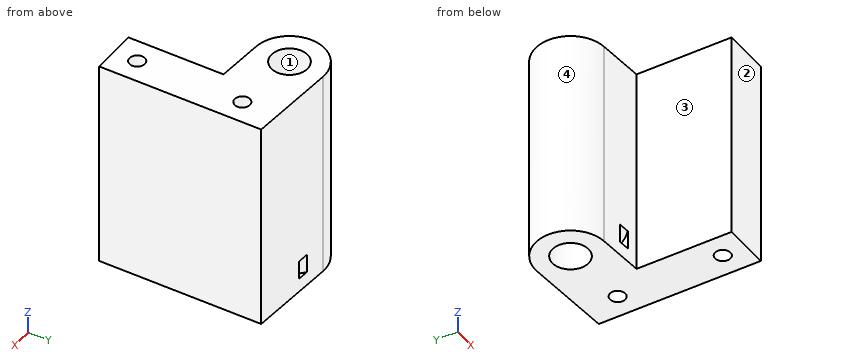
```python
from build123d import *

# Parameters (mm, degrees)
BOSS_EXTRUDE1_DEPTH   = 45
CUT_EXTRUDE1_START    = -5
CUT_EXTRUDE1_DEPTH    = 2
M4X0_7_TAPPED_HOLE1_D = 3.3
SKETCH5_R             = 7.5
BOSS_EXTRUDE2_DEPTH   = 45
SKETCH6_R             = 3.875
CUT_EXTRUDE2_DEPTH    = 46


with BuildPart() as part:
    # Sketch1 → Boss-Extrude1 (new body)
    with BuildSketch(Plane.XY):
        with BuildLine():
            Line((-182.516015687, 162.517772537), (-172.5, 161.827012834))
            Line((-172.5, 161.827012834), (-172.5, 141.5))
            Line((-172.5, 141.5), (-162.5, 141.5))
            Line((-162.5, 141.5), (-162.5, 176.172987166))
            Line((-162.5, 176.172987166), (-181.483984313, 177.482227463))
            ThreePointArc((-181.483984313, 177.482227463), (-174.517772537, 169.483984313), (-182.516015687, 162.517772537))
        make_face()
    extrude(amount=BOSS_EXTRUDE1_DEPTH)

    # Sketch2 → Cut-Extrude1 (cut, symmetric)
    with BuildSketch(Plane(origin=(0, 0, 0), x_dir=(-1, 0, 0), z_dir=(0, 0, -1)).offset(CUT_EXTRUDE1_START)):
        with BuildLine():
            ThreePointArc((176.520836095, 177.139941379), (173.021327044, 169.380781175), (177.552867469, 162.175486453))
            ThreePointArc((177.552867469, 162.175486453), (177.834315887, 161.15284928), (176.811678714, 160.871400862))
            ThreePointArc((176.811678714, 160.871400862), (171.524881552, 169.277578038), (175.60764211, 178.329931609))
            ThreePointArc((175.60764211, 178.329931609), (176.659234217, 178.191533486), (176.520836095, 177.139941379))
        make_face()
    extrude(amount=CUT_EXTRUDE1_DEPTH, both=True, mode=Mode.SUBTRACT)

    # M4x0.7 Tapped Hole1 (through all)
    with Locations(Plane.XY.offset(45)):
        with Locations((-167.5, 169), (-167.5, 146.5)):
            Hole(M4X0_7_TAPPED_HOLE1_D / 2)

    # Sketch5 → Boss-Extrude2 (add, through all)
    with BuildSketch(Plane.XY.offset(45)):
        with Locations((-182, 170)):
            Circle(SKETCH5_R)
    extrude(amount=-BOSS_EXTRUDE2_DEPTH)

    # Sketch6 → Cut-Extrude2 (cut, through all)
    with BuildSketch(Plane.XY.offset(45)):
        with Locations((-182, 170)):
            Circle(SKETCH6_R)
    extrude(amount=-CUT_EXTRUDE2_DEPTH, mode=Mode.SUBTRACT)


solid = part.part
```
For this review, take the finished solid that the model builds, in its own axes (mm). Face numbers are marked on the shaded views. Coordinates: 2 decimals unless noted, no trailing zeros. Loops run counter-clockwise (first coordinate to the right, second up) from the corner with the lowest first, then second, coordinate; pieces in that order, holes last. Notation, with made-up numbers: (-17.5, 62) -> (-9.5, 62) arc R21 cw to (-9.5, 93) -> close; hole circle Ø2 at (67, 20). An arc over 180 degrees is marked (long way). Return JSON: item names as keys, results as strings. Group by question number.
(1) Consider section A-A, the plane y = 169. Give the boundary of the cut face in (x, z), plus the area to 3 significant figures.
(2) Consider section D-D, the plane y = 164. Give the boundary of the cut face in (x, z).
(3) Consider section B-B, the plane x = -182. Give the boundary of the cut face in (y, z) (3 decimals), plus the area to 3 significant figures.
(4) Consider section C-C, the plane z = 8. Give the boundary of the cut face in (x, y) (3 decimals), plus the area to 3 significant figures.
(5) For pin 1 Ø4 at (x, z) = (-181.5, 24) entering from -Y; pin 2 Ø3 at (x, y) = (-167.5, 146.5) entering from +Z; pin 3 Ø16.5 at (y, z) = (156.5, 18.5) entering from -X; pin 4 Ø5 at (x, z) = (-171.5, 25.5) entering from +Y, all flat-tipped, find the tip position at first contact; note any pin that passes through.
(6) To check wall thickness, follow L1, parallel to Y at x = -168.75, z = 6; L2, parallel to X at y = 146.5, z = 26.5; L3, parallel to Y at x = -167.5, z = 30. State the ranges of each line that lie inside material, in increasing order.
(7) Mouldability with a two-part tool opening along Y and no side actions: class the marked faces 1, 2, 3 and 4 as pulls with the +Y half, pulls with the -Y half, needs draft (parallel to the pull), parting line crosses it, or undercut.
Results below:
{
 "1": {"outline": "(-189.43, 0) -> (-185.74, 0) -> (-185.74, 45) -> (-189.43, 45) -> close; (-178.26, 0) -> (-169.15, 0) -> (-169.15, 45) -> (-178.26, 45) -> close; (-165.85, 0) -> (-162.5, 0) -> (-162.5, 45) -> (-165.85, 45) -> close; hole (-173.06, 3) -> (-171.55, 3) -> (-171.55, 7) -> (-173.06, 7) -> close", "area": "721 mm2"},
 "2": {"outline": "(-186.5, 0) -> (-162.5, 0) -> (-162.5, 45) -> (-186.5, 45) -> close; hole (-175.29, 3) -> (-173.38, 3) -> (-173.38, 7) -> (-175.29, 7) -> close"},
 "3": {"outline": "(162.482, 0) -> (166.125, 0) -> (166.125, 45) -> (162.482, 45) -> close; (173.875, 0) -> (177.5, 0) -> (177.5, 45) -> (173.875, 45) -> close", "area": "327 mm2"},
 "4": {"outline": "(-182.516, 162.518) -> (-172.5, 161.827) -> (-172.5, 141.5) -> (-162.5, 141.5) -> (-162.5, 176.173) -> (-181.484, 177.482) arc R7.5 ccw to start; hole circle Ø7.75 at (-182, 170); hole circle Ø3.3 at (-167.5, 146.5); hole circle Ø3.3 at (-167.5, 169)", "area": "517 mm2"},
 "5": {"pin 1": "stops at y = 162.31", "pin 2": "passes through", "pin 3": "stops at x = -187.36", "pin 4": "stops at y = 176.97"},
 "6": {"L1": "y = 141.5 to 145.42, 147.58 to 167.92, 170.08 to 176.6", "L2": "x = -172.5 to -169.15, -165.85 to -162.5", "L3": "y = 141.5 to 144.85, 148.15 to 167.35, 170.65 to 176.52"},
 "7": {"face 1": "undercut", "face 2": "pulls with the -Y half", "face 3": "needs draft", "face 4": "parting line crosses it"}
}
